The listing builds one solid part. Answer for the finished solid, in the listing's coordinates (mm). A direction names the side the tool comes from. Coordinates: 2 decimals unless noted, no trailing zeros. Order: outer loops, then holes, each group sorted by start corner. A loop starts at its lowest first (then second) coordinate and runs counter-clockwise, first axis right, second up. Notation, with made-up numbers: (-16.75, -30.5) - (30.25, -30.5) arc R15 ccw to (30.25, -2.5) - close; hole circle Ø10 at (23.25, -27). An arc over 180 degrees is marked (long way). Use a Markdown table: item, result. Add a question column.
Item 1: For faces 4 (the flat face through (-5, 4.25, -4)), 5 (the cylindrical face through (9.699, 4.563, -7.215)), 6 (the cylindrical face through (4.35, 2.07, 3.56)), determine the directions among +Z, -Z, +X, -X, +Y, -Y from which every point of the face is accessible in a straight line to the end or side of a thin tool.
Item 2: The mould has two halves that part along X. Classify faces 1 (the flat face through (10, 4, 0)), 2 (the cylindrical face through (-9.715, 4.563, 7.199)), 3 (the flat face through (5, 4.25, -4)): released by +X, released by -X, zero draft, split by the parting line, or undercut.
Item 3: The part is cut by section A-A, the plane z = -1.5. Give the vertices of the cut face in (x, y).
Item 4: Find the intervals of material crossed by line 1 along Y through (x, z) = (-5, 3.5); line 2 along X through (y, z) = (5.75, 6.25); line 3 along Z through (x, y) = (7.5, 6), in increasing order.
Item 5: The part is cut by section D-D, the plane y = 3. Give the vertices of the cut face in (x, z).
Item 6: The part is cut by section C-C, the plane y = 6.5. Give the vertices of the cut face in (x, z), then the cut area to 3 significant figures.
Item 7: The part is cut by section B-B, the plane y = 4.5. Give the vertices of the cut face in (x, z).
Item 8: A flat-ended cylindrical pin translates along its axis: P1, Ø1.8, axis at x = 4, y = 5, coming from the +Z side. Find the tip coordinate at first contact, or state that the pin passes through.
from build123d import *

# Parameters (mm, degrees)
SKETCH1_W           = 20
SKETCH1_H           = 15
BOSS_EXTRUDE1_DEPTH = 10
SKETCH4_R           = 3
CUT_EXTRUDE1_DEPTH  = 8
CUT_EXTRUDE2_DEPTH  = 8
FILLET1_R           = 1


with BuildPart() as part:
    # Sketch1 → Boss-Extrude1 (new body)
    with BuildSketch(Plane(origin=(0, 0, 0), x_dir=(1, 0, 0), z_dir=(0, 1, 0))):
        Rectangle(SKETCH1_W, SKETCH1_H)
    extrude(amount=BOSS_EXTRUDE1_DEPTH)

    # Sketch4 → Cut-Extrude1 (cut)
    with BuildSketch(Plane.XY.offset(7.5)):
        with Locations((5, 5)):
            Circle(SKETCH4_R)
    cut_extrude1 = extrude(amount=-CUT_EXTRUDE1_DEPTH, mode=Mode.SUBTRACT)

    # Sketch6 → Cut-Extrude2 (cut, through all)
    with BuildSketch(Plane.XY.offset(-0.5)):
        with BuildLine():
            Line((3.75, 5.75), (6.25, 5.75))
            ThreePointArc((6.25, 5.75), (7, 5), (6.25, 4.25))
            Line((6.25, 4.25), (3.75, 4.25))
            ThreePointArc((3.75, 4.25), (3, 5), (3.75, 5.75))
        make_face()
    cut_extrude2 = extrude(amount=-CUT_EXTRUDE2_DEPTH, mode=Mode.SUBTRACT)

    # Mirror1: Cut-Extrude1, Cut-Extrude2 across plane
    add(cut_extrude1.mirror(Plane(origin=(0, 0, 0), x_dir=(0, 0, 1), z_dir=(1, 0, 0))), mode=Mode.SUBTRACT)
    add(cut_extrude2.mirror(Plane(origin=(0, 0, 0), x_dir=(0, 0, 1), z_dir=(1, 0, 0))), mode=Mode.SUBTRACT)

    # Fillet1
    fillet1_edges = [part.edges().sort_by_distance(p)[0] for p in [
        (-10, 10, 0),
        (0, 10, 7.5),
        (10, 10, 0),
        (0, 10, -7.5),
        (10, 5, 7.5),
        (-10, 5, 7.5),
        (-10, 5, -7.5),
        (10, 5, -7.5),
    ]]
    fillet(fillet1_edges, radius=FILLET1_R)


solid = part.part
Solution:
| question | item | result |
|---|---|---|
| 1 | face 4 | +Z, -Z |
| 1 | face 5 | -Z, +X, +Y, -Y |
| 1 | face 6 | +Z |
| 2 | face 1 | released by +X |
| 2 | face 2 | released by -X |
| 2 | face 3 | undercut |
| 3 | outline | (-10, 0) - (10, 0) - (10, 9) arc R1 ccw to (9, 10) - (-9, 10) arc R1 ccw to (-10, 9) - close; hole (-6.25, 4.25) - (-3.75, 4.25) arc R0.75 ccw to (-3.75, 5.75) - (-6.25, 5.75) arc R0.75 ccw to start; hole (3.75, 4.25) - (6.25, 4.25) arc R0.75 ccw to (6.25, 5.75) - (3.75, 5.75) arc R0.75 ccw to start |
| 4 | line 1 | y = 0 to 2, 8 to 10 |
| 4 | line 2 | x = -10 to -7.9, -2.1 to 2.1, 7.9 to 10 |
| 4 | line 3 | z = -7.5 to -0.5 |
| 5 | outline | (-10, -6.5) arc R1 ccw to (-9, -7.5) - (9, -7.5) arc R1 ccw to (10, -6.5) - (10, 6.5) arc R1 ccw to (9, 7.5) - (7.24, 7.5) - (7.24, -0.5) - (2.76, -0.5) - (2.76, 7.5) - (-2.76, 7.5) - (-2.76, -0.5) - (-7.24, -0.5) - (-7.24, 7.5) - (-9, 7.5) arc R1 ccw to (-10, 6.5) - close |
| 6 | outline | (-10, -6.5) arc R1 ccw to (-9, -7.5) - (9, -7.5) arc R1 ccw to (10, -6.5) - (10, 6.5) arc R1 ccw to (9, 7.5) - (7.6, 7.5) - (7.6, -0.5) - (2.4, -0.5) - (2.4, 7.5) - (-2.4, 7.5) - (-2.4, -0.5) - (-7.6, -0.5) - (-7.6, 7.5) - (-9, 7.5) arc R1 ccw to (-10, 6.5) - close |
| 6 | area | 216 mm2 |
| 7 | outline | (-10, -6.5) arc R1 ccw to (-9, -7.5) - (-6.81, -7.5) - (-6.81, -0.5) - (-7.96, -0.5) - (-7.96, 7.5) - (-9, 7.5) arc R1 ccw to (-10, 6.5) - close; (-3.19, -7.5) - (3.19, -7.5) - (3.19, -0.5) - (2.04, -0.5) - (2.04, 7.5) - (-2.04, 7.5) - (-2.04, -0.5) - (-3.19, -0.5) - close; (6.81, -7.5) - (9, -7.5) arc R1 ccw to (10, -6.5) - (10, 6.5) arc R1 ccw to (9, 7.5) - (7.96, 7.5) - (7.96, -0.5) - (6.81, -0.5) - close |
| 8 | P1 | stops at z = -0.5 |
